```python
from build123d import *

# Parameters (mm, degrees)
F1_DEPTH = 10


with BuildPart() as f1:
    # F0 (on Front) → F1 (new body)
    with BuildSketch(Plane.XZ):
        with BuildLine():
            Line((-135, 10), (0, 10))
            Line((0, 10), (0, 60))
            ThreePointArc((0, 60), (-73.4846922835, 81.7524834709), (-123.2882800594, 140))
            Line((-123.2882800594, 140), (-185, 140))
            Line((-185, 140), (-185, 0))
            Line((-185, 0), (-135, 0))
            Line((-135, 0), (-135, 10))
        make_face()
        with BuildLine():
            Line((135, 10), (135, 0))
            Line((135, 0), (185, 0))
            Line((185, 0), (185, 140))
            Line((185, 140), (123.2882800594, 140))
            ThreePointArc((123.2882800594, 140), (73.4846922835, 81.7524834709), (0, 60))
            Line((0, 60), (0, 10))
            Line((0, 10), (135, 10))
        make_face()
    extrude(amount=F1_DEPTH)


solid = f1.part
```
Geometry: final body of the model. Coordinates: model frame, mm. A direction names the side the tool comes from. Coordinates: 2 decimals unless noted, no trailing zeros. Loops run counter-clockwise (first coordinate to the right, second up) from the corner with the lowest first, then second, coordinate; pieces in that order, holes last. Notation, with made-up numbers: M 65,22 L 105,22 A17 ccw 105,38 Z; hole C -29.5,63.5 d6. An arc over 180 degrees is marked long. Put each result on its own line as item: value.
(1) Cut plane C-C on z = 115. Return the cut outline in (x, y).
Answer sheet:
outline: M -185,-10 L -108.74,-10 L -108.74,0 L -185,0 Z; M 108.74,-10 L 185,-10 L 185,0 L 108.74,0 Z
(2) First-contact query: pin 1 (2 mm diameter, centred on x = -103, z = 108.5, fed in from -Y); pin 2 (5 mm diameter, centred on x = -111.5, y = -1.5, fed in from -Z). Flat tips, straight axial feed; report the tip coordinate or a pass-through.
Answer sheet:
pin 1: stops at y = -10
pin 2: stops at z = 10
(3) Cut plane D-D on x = 32.5. Return the cut outline in (y, z).
Answer sheet:
outline: M -10,10 L 0,10 L 0,63.97 L -10,63.97 Z
(4) Cut plane B-B on y = -6.5. Return the cut outline in (x, z).
Answer sheet:
outline: M -185,0 L -135,0 L -135,10 L 135,10 L 135,0 L 185,0 L 185,140 L 123.29,140 A135 cw -123.29,140 L -185,140 Z
(5) Cut plane A-A on z = 101. Return the cut outline in (x, y), then the cut area to 3 significant figures.
Answer sheet:
outline: M -185,-10 L -96.9,-10 L -96.9,0 L -185,0 Z; M 96.9,-10 L 185,-10 L 185,0 L 96.9,0 Z
area: 1,760 mm^2
(6) Material intervals for probe 1 along Z at (x, y) = (129, -0.75); probe 2 along X at (y, z) = (-5.75, 129); probe 3 along X at (y, z) = (-1.75, 125), sorted ascending.
Answer sheet:
probe 1: z = 10 to 140
probe 2: x = -185 to -117.77, 117.77 to 185
probe 3: x = -185 to -115.43, 115.43 to 185
(7) Access query for faces 4 (the face through (155, -5, 140)), 5 (the face through (135, -5, 5)). Directions: +Z, -Z, +X, -X, +Y, -Y. A direction counts if a zero-diameter tool reaches every point of the face in a straight line with its end or side. Return the directions, or none.
Answer sheet:
face 4: +Z, +X, -X, +Y, -Y
face 5: -Z, +Y, -Y
(8) Draft query along X for faces 1 (the face through (-185, -5, 71)), 2 (the face through (-160, -5, 0)), 3 (the face through (-135, -5, 5)). Return one class per face: pulls with the +X half, pulls with the -X half, needs draft (parallel to the pull), parting line crosses it, or undercut.
Answer sheet:
face 1: pulls with the -X half
face 2: needs draft
face 3: undercut
